```python
from build123d import *

# Parameters (mm, degrees)
ENL_V_MAT_EXTRU_1_DEPTH      = 31.033314835
ENL_V_MAT_EXTRU_1_DEPTH_BACK = 31.033314835
ESQUISSE2_R                  = 5.1
ENL_V_MAT_EXTRU_2_DEPTH      = 26.670995306
ENL_V_MAT_EXTRU_2_DEPTH_BACK = 26.670995306
ESQUISSE3_R                  = 1
ESQUISSE4_R                  = 1.65
ENL_V_MAT_EXTRU_3_DEPTH      = 26.670995306


with BuildPart() as part:
    # Esquisse1 → Révolution1 (revolve)
    with BuildSketch(Plane.XY):
        Polygon((9, 0), (9, 17), (7, 15), (-7, 15), (-9, 17), (-9, 0), align=None)
    revolve(axis=Axis((9, 0, 0), (-1, 0, 0)))

    # Esquisse2 → Enlèv. mat.-Extru.1 (cut, two sides: drawn at the far end of the back side and taken through both)
    with BuildSketch(Plane.ZY.offset(9).offset(-ENL_V_MAT_EXTRU_1_DEPTH_BACK)):
        Circle(ESQUISSE2_R)
    extrude(amount=ENL_V_MAT_EXTRU_1_DEPTH + ENL_V_MAT_EXTRU_1_DEPTH_BACK, mode=Mode.SUBTRACT)

    # Esquisse3 → Enlèv. mat.-Extru.2 (cut, two sides: drawn at the far end of the back side and taken through both)
    with BuildSketch(Plane.XY.offset(-ENL_V_MAT_EXTRU_2_DEPTH_BACK)):
        with Locations((-5, 12)):
            Circle(ESQUISSE3_R)
    extrude(amount=ENL_V_MAT_EXTRU_2_DEPTH + ENL_V_MAT_EXTRU_2_DEPTH_BACK, mode=Mode.SUBTRACT)

    # Esquisse4 → Enlèv. mat.-Extru.3 (cut, through all)
    with BuildSketch(Plane.XY):
        Circle(ESQUISSE4_R)
    extrude(amount=-ENL_V_MAT_EXTRU_3_DEPTH, mode=Mode.SUBTRACT)


solid = part.part
```
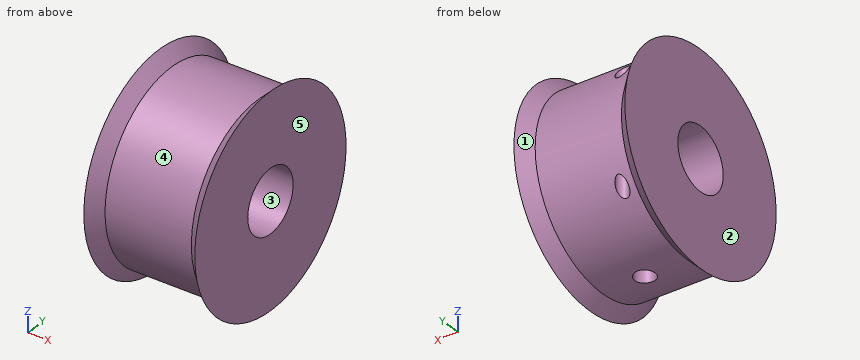
CAD build for the part. Positions are in the model's coordinates, mm. Face numbers are marked on the shaded views. A direction names the side the tool comes from. Coordinates: 2 decimals unless noted, no trailing zeros. Order: outer loops, then holes, each group sorted by start corner. A loop starts at its lowest first (then second) coordinate and runs counter-clockwise, first axis right, second up. Notation, with made-up numbers: (63, 86) - (82, 86) arc R4 ccw to (82, 91) - close; hole circle Ø10 at (57, 19.5). An arc over 180 degrees is marked (long way). Use a Markdown table: item, result. Add a question column.
(1) Saw through at A-A (z = 0). Give the cut face in (x, y), then the cut area to 3 significant figures.
(2) Drill centre lines: line 1 along X through (y, z) = (0, -9.5); line 2 along Z through (x, y) = (-7.5, 4.5); line 3 along Y through (x, z) = (3.5, 11). Where is each one in solid material? Low to high. Write a range as [from, to].
(3) Flat gauge pins, fed straight in: pin 1 (3 mm diameter, centred on x = -4, z = 1, fed in from +Y); pin 2 (1.5 mm diameter, centred on x = 2, z = 10, fed in from +Y); pin 3 (1.5 mm diameter, centred on x = 2.5, y = -10.5, fed in from +Z). Where does each tip first touch, or does it go through?
(4) Saw through at D-D (x = 4.5). Give the cut face in (y, z).
(5) Which spindle directions (+Z, -Z, +X, -X, +Y, -Y) get a long thin tool onto all of the face, cutting with end or side? Do the marked faces 4 and 5. Say none if no direction does.
(6) Saw through at B-B (y = 0). Give the cut face in (x, z).
(7) Saw through at C-C (x = -5). Give the cut face in (y, z), then the cut area to 3 significant figures.
(8) Pull direction X, two halves, no side cores. Call the marked faces 1, 2 and 3: +X half, -X half, draft (parallel to the pull), parting line (faces both ways), or undercut.
Solved:
| question | item | result |
|---|---|---|
| 1 | outline | (-9, -17) - (-7, -15) - (7, -15) - (9, -17) - (9, -5.1) - (-9, -5.1) - close; (-9, 5.1) - (9, 5.1) - (9, 17) - (7, 15) - (-7, 15) - (-9, 17) - close; hole circle Ø2 at (-5, 12) |
| 1 | area | 361 mm² |
| 2 | line 1 | x = [-9, -1.65], [1.65, 9] |
| 2 | line 2 | z = [-14.83, -2.4], [2.4, 14.83] |
| 2 | line 3 | y = [-10.2, 10.2] |
| 3 | pin 1 | stops at y = 15 |
| 3 | pin 2 | stops at y = 11.81 |
| 3 | pin 3 | stops at z = 11.4 |
| 4 | outline | circle Ø30 at (0, 0); hole circle Ø10.2 at (0, 0) |
| 5 | face 4 | none |
| 5 | face 5 | +Z, -Z, +X, +Y, -Y |
| 6 | outline | (-9, -17) - (-7, -15) - (-1.65, -15) - (-1.65, -5.1) - (-9, -5.1) - close; (-9, 5.1) - (9, 5.1) - (9, 17) - (7, 15) - (-7, 15) - (-9, 17) - close; (1.65, -15) - (7, -15) - (9, -17) - (9, -5.1) - (1.65, -5.1) - close |
| 7 | outline | (11, -10.2) - (11, 10.2) arc R15 ccw (long way) to start; (13, -7.48) arc R15 ccw to (13, 7.48) - close; hole circle Ø10.2 at (0, 0) |
| 7 | area | 589 mm² |
| 8 | face 1 | undercut |
| 8 | face 2 | -X half |
| 8 | face 3 | draft |
